Part model, mm, in its own coordinate system. Give positions to 0.01 mm unless a question says otherwise; leave off trailing zeros. Write each loop counter-clockwise with the first axis right and the second up, starting at its lowest first coordinate (ties: lowest second). Pieces come first, ordered by that corner, then holes.
```python
from build123d import *
from OCP.BRepFilletAPI import BRepFilletAPI_MakeChamfer

# Parameters (mm, degrees)
SKETCH_1_R      = 9.5
EXTRUDE_1_DEPTH = 4
CHAMFER_1_SIZE  = 0.5
CHAMFER_1_SIZE2 = 0.133974596


with BuildPart() as part:
    # 草图1 → 凸台-拉伸1 (new body)
    with BuildSketch(Plane(origin=(0, 0, 0), x_dir=(1, 0, 0), z_dir=(0, 1, 0))):
        Polygon((6.25, 10.825317547), (-6.25, 10.825317547), (-12.5, 0), (-6.25, -10.825317547), (6.25, -10.825317547), (12.5, 0), align=None)
        with Locations(Location((0, 0, 0), (0, 0, 270))):
            Circle(SKETCH_1_R, mode=Mode.SUBTRACT)
    extrude(amount=EXTRUDE_1_DEPTH)

    # 草图2 → 切除-旋转2 (revolve, cut)
    with BuildSketch(Plane.XY):
        Polygon((11, 4), (12.5, 4), (12.5, 3.5), align=None)
        Polygon((12.5, 0.5), (12.5, 0), (11, 0), align=None)
    revolve(axis=Axis((0, 0, 0), (0, 1, 0)), mode=Mode.SUBTRACT)

    # 倒角1: one chamfer whose edges measure the first distance from different faces: ONE call of the kernel's chamfer builder (chamfer() names one face for all edges)
    chamfer_1_edges_1 = [part.edges().sort_by_distance(p)[0] for p in [
        (0, 0, -9.5),
    ]]
    chamfer_1_side_1 = [part.faces().sort_by_distance(p)[0] for p in [
        (0, 2, -9.5),
    ]]
    chamfer_1_edges_2 = [part.edges().sort_by_distance(p)[0] for p in [
        (0, 4, -9.5),
    ]]
    chamfer_1_side_2 = [part.faces().sort_by_distance(p)[0] for p in [
        (5.345666757, 4, -9.258966423),
    ]]
    chamfer_1 = BRepFilletAPI_MakeChamfer(part.part.solid().wrapped)
    for e in chamfer_1_edges_1:
        chamfer_1.Add(CHAMFER_1_SIZE, CHAMFER_1_SIZE2, e.wrapped, chamfer_1_side_1[0].wrapped)  # the first distance lies on this face
    for e in chamfer_1_edges_2:
        chamfer_1.Add(CHAMFER_1_SIZE, CHAMFER_1_SIZE2, e.wrapped, chamfer_1_side_2[0].wrapped)  # the first distance lies on this face
    add(Compound.cast(chamfer_1.Shape()), mode=Mode.REPLACE)


solid = part.part
```
1) Wall check: L1, parallel to Z at x = 2, y = 0.8; L2, parallel to Z at x = 3, y = 0.6; L3, parallel to X at y = 3.6, z = -6.25. Give the ranges that are in metal, low to high.
Answers follow:
L1: z = -10.83 to -9.29, 9.29 to 10.83
L2: z = -10.83 to -9.01, 9.01 to 10.83
L3: x = -8.89 to -7.15, 7.15 to 8.89
2) Two-plate mould, pull along Z, no slides. Class faces 1 (the face through (-11.406, 3.865, -0.055)), 2 (the face through (-5.67, 0.14, -9.92)), 3 (the face through (-5.78, 2.16, -7.54)), 4 (the face through (-5.761, 0.142, 9.868)): +Z half, -Z half, draft (parallel to the pull), parting line (faces both ways), or undercut.
Answers follow:
face 1: parting line
face 2: -Z half
face 3: undercut
face 4: +Z half
3) Pin check, flat tips, straight feed: pin 1 Ø1.5 at (y, z) = (3, 3.5) entering from +X; pin 2 Ø5 at (x, z) = (4, 3) entering from -Y; pin 3 Ø5 at (x, z) = (9.5, -2.5) entering from -Y. Stop position of each tip, or through.
Answers follow:
pin 1: stops at x = 10.91
pin 2: passes through
pin 3: stops at y = 0
4) Saw through at B-B, the plane y = 3.1. Write the cut outline in (x, z).
Answers follow:
outline: (-12.5, 0) - (-6.25, -10.83) - (6.25, -10.83) - (12.5, 0) - (6.25, 10.83) - (-6.25, 10.83) - close; hole circle Ø19 at (0, 0)
5) Saw through at A-A, the plane x = 0. Write the cut outline in (y, z), then the cut area to 3 significant figures.
Answers follow:
outline: (0, -10.83) - (4, -10.83) - (4, -10) - (3.87, -9.5) - (0.5, -9.5) - (0, -9.63) - close; (0, 9.63) - (0.5, 9.5) - (3.87, 9.5) - (4, 10) - (4, 10.83) - (0, 10.83) - close
area: 10.5 mm2
